Check sheet for the modelled part. Datum: model origin and axes. Units: mm. Face numbers are marked on the shaded views. A direction names the side the tool comes from. Give positions to 0.01 mm unless a question says otherwise; leave off trailing zeros. Order: outer loops, then holes, each group sorted by start corner. A loop starts at its lowest first (then second) coordinate and runs counter-clockwise, first axis right, second up.
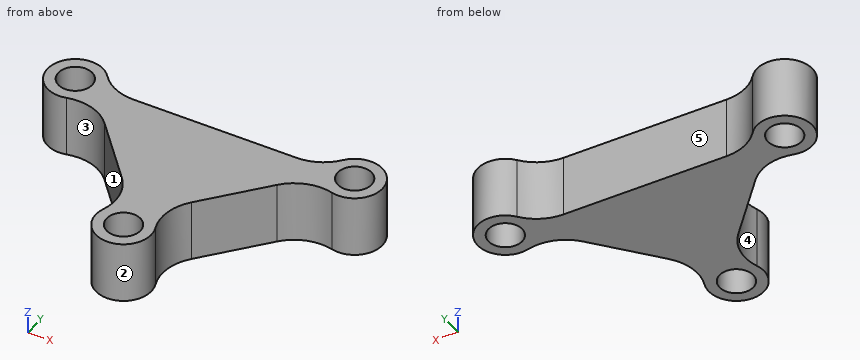
```python
from build123d import *

# Parameters (mm, degrees)
ESQUISSE2_R        = 3
ESQUISSE2_R_2      = 1.825
BOSS_EXTRU_1_DEPTH = 6.64
CONG_1_R           = 5


with BuildPart() as part:
    # Esquisse2 → Boss.-Extru.1 (new body)
    # profile 1 of 4: a face of its own
    with BuildSketch(Plane.XY):
        with Locations((-15, 10)):
            Circle(ESQUISSE2_R)
        with Locations(Location((-15, 10, 0), (0, 0, 180))):
            Circle(ESQUISSE2_R_2, mode=Mode.SUBTRACT)
    # profile 2 of 4: a face of its own
    with BuildSketch(Plane.XY):
        with Locations((15, 10)):
            Circle(ESQUISSE2_R)
        with Locations(Location((15, 10, 0), (0, 0, 180))):
            Circle(ESQUISSE2_R_2, mode=Mode.SUBTRACT)
    # profile 3 of 4: a face of its own
    with BuildSketch(Plane.XY):
        with Locations((0, -6.825)):
            Circle(ESQUISSE2_R)
        with Locations(Location((0, -6.825, 0), (0, 0, 180))):
            Circle(ESQUISSE2_R_2, mode=Mode.SUBTRACT)
    # profile 4 of 4: a face of its own
    with BuildSketch(Plane.XY):
        Polygon((-13.175, 10), (13.175, 10), (0, -5), align=None)
    extrude(amount=BOSS_EXTRU_1_DEPTH)

    # Congé1
    cong_1_edges = [part.edges().sort_by_distance(p)[0] for p in [
        (-12.208908932, 8.900086071, 3.32),
        (-12, 10, 3.32),
        (12, 10, 3.32),
        (12.208908932, 8.900086071, 3.32),
        (0.908352526, -3.965822551, 3.32),
        (-0.908352526, -3.965822551, 3.32),
    ]]
    fillet(cong_1_edges, radius=CONG_1_R)


solid = part.part
```
(1) Set-up check for the marked faces 4 and 5: record each of +Z, -Z, +X, -X, +Y, -Y from which the full face is reachable in a straight line by a thin tool's end or side.
Response values:
face 4: +Z, -Z, -X
face 5: +Z, -Z, +Y
(2) Release check for a two-part mould opening along X. For the marked faces 1, 2 and 3 record: released by +X, released by -X, zero draft, split by the parting line, or undercut.
Response values:
face 1: released by -X
face 2: split by the parting line
face 3: undercut
(3) Cross-section at D-D on x = 0. Enter the section's corners in (y, z) (3 decimals).
Response values:
outline: (-9.825, 0) - (-8.65, 0) - (-8.65, 6.64) - (-9.825, 6.64) - close; (-5, 0) - (10, 0) - (10, 6.64) - (-5, 6.64) - close
(4) Cross-section at C-C on z = 2.5. Enter the section's corners in (x, y) (3 decimals), then the cut area to 3 significant figures.
Response values:
outline: (-14.258, 7.093) arc R5 cw to (-9.265, 5.548) - (-3.742, -0.739) arc R5 cw to (-2.812, -5.78) arc R3 ccw (long way) to (2.812, -5.78) arc R5 cw to (3.742, -0.739) - (9.265, 5.548) arc R5 cw to (14.258, 7.093) arc R3 ccw (long way) to (12.658, 11.875) arc R5 cw to (8.755, 10) - (-8.755, 10) arc R5 cw to (-12.658, 11.875) arc R3 ccw (long way) to start; hole circle Ø3.65 at (-15, 10); hole circle Ø3.65 at (0, -6.825); hole circle Ø3.65 at (15, 10)
area: 262 mm2
(5) Gauge pin test, flat ends, axial feed: pin 1 Ø2 at (x, z) = (-0.5, 3.5) entering from +Y; pin 2 Ø3 at (x, z) = (-9.5, 2) entering from -Y; pin 3 Ø2 at (x, y) = (0, -6.825) entering from -Z. Record the tip position at first contact, or that the pin passes through.
Response values:
pin 1: stops at y = 10
pin 2: stops at y = 4.11
pin 3: passes through
(6) Cross-section at A-A on x = -15. Enter the section's corners in (y, z) (3 decimals), then the cut area to 3 significant figures.
Response values:
outline: (7, 0) - (8.175, 0) - (8.175, 6.64) - (7, 6.64) - close; (11.825, 0) - (13, 0) - (13, 6.64) - (11.825, 6.64) - close
area: 15.6 mm2
(7) Material ranges on L1, parallel to Y at x = 0, z = 4.25 (3 decimals); L2, parallel to Y at x = 15, z = 2.5 (3 decimals); L3, parallel to X at y = -6.75, z = 1.5, recorded low to high.
Response values:
L1: y = -9.825 to -8.65, -5 to 10
L2: y = 7 to 8.175, 11.825 to 13
L3: x = -3 to -1.82, 1.82 to 3
(8) Cross-section at B-B on y = 11. Enter the section's corners in (x, z) (3 decimals).
Response values:
outline: (-17.828, 0) - (-16.527, 0) - (-16.527, 6.64) - (-17.828, 6.64) - close; (-13.473, 0) - (-11.755, 0) - (-11.755, 6.64) - (-13.473, 6.64) - close; (11.755, 0) - (13.473, 0) - (13.473, 6.64) - (11.755, 6.64) - close; (16.527, 0) - (17.828, 0) - (17.828, 6.64) - (16.527, 6.64) - close
